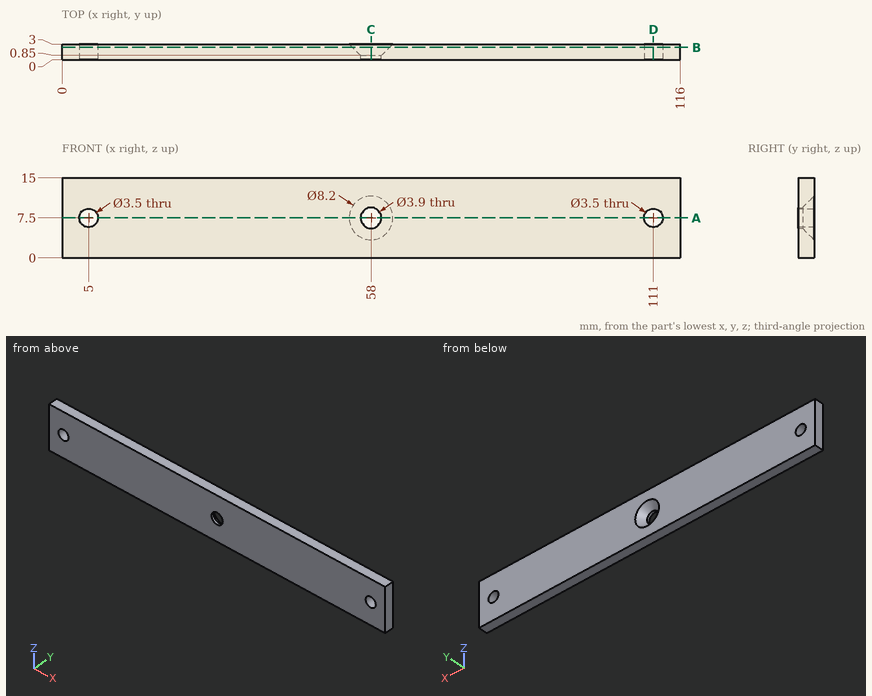
Geometry check sheet. Reference: drawing and pictorial views, mm from the part's lowest x, y, z. Coordinates: 2 decimals unless noted, no trailing zeros. Order: outer loops, then holes, each group sorted by start corner. A loop starts at its lowest first (then second) coordinate and runs counter-clockwise, first axis right, second up.
1. Sectioned sample at B-B, the plane y = 2.35. Record the cut outline in (x, z), and give its area (3 significant figures).
Results found:
outline: (0, 0) - (116, 0) - (116, 15) - (0, 15) - close; hole circle Ø3.5 at (5, 7.5); hole circle Ø6.9 at (58, 7.5); hole circle Ø3.5 at (111, 7.5)
area: 1,680 mm2
2. Sectioned sample at A-A, the plane z = 7.5. Record the cut outline in (x, y).
Results found:
outline: (0, 0) - (3.25, 0) - (3.25, 3) - (0, 3) - close; (6.75, 0) - (56.05, 0) - (56.05, 0.85) - (53.9, 3) - (6.75, 3) - close; (59.95, 0) - (109.25, 0) - (109.25, 3) - (62.1, 3) - (59.95, 0.85) - close; (112.75, 0) - (116, 0) - (116, 3) - (112.75, 3) - close
3. Sectioned sample at C-C, the plane x = 58. Record the cut outline in (y, z).
Results found:
outline: (0, 0) - (3, 0) - (3, 3.4) - (0.85, 5.55) - (0, 5.55) - close; (0, 9.45) - (0.85, 9.45) - (3, 11.6) - (3, 15) - (0, 15) - close
4. Scan lines: line 1 (X direction, y = 0.6, z = 7.5); line 2 (X direction, y = 1.9, z = 8.5); line 3 (Z direction, x = 58, y = 0.5). Record each from-to range of solid material in increasing order.
Results found:
line 1: x = 0 to 3.25, 6.75 to 56.05, 59.95 to 109.25, 112.75 to 116
line 2: x = 0 to 3.56, 6.44 to 55.17, 60.83 to 109.56, 112.44 to 116
line 3: z = 0 to 5.55, 9.45 to 15
5. Sectioned sample at D-D, the plane x = 111. Record the cut outline in (y, z).
Results found:
outline: (0, 0) - (3, 0) - (3, 5.75) - (0, 5.75) - close; (0, 9.25) - (3, 9.25) - (3, 15) - (0, 15) - close
